The model under review builds one solid part; all positions refer to its coordinate system, in mm. A direction names the side the tool comes from. Round coordinates to 2 decimals unless told otherwise and drop trailing zeros. Loops run counter-clockwise (first coordinate to the right, second up) from the corner with the lowest first, then second, coordinate; pieces in that order, holes last. Notation, with made-up numbers: M -15.75,15 L 27.25,15 A19 cw 27.25,32 Z; hole C 72.5,80.5 d7. An arc over 180 degrees is marked long. One line per question, with ' | ' between items.
from build123d import *

# Parameters (mm, degrees)
BOSS_EXTRUDE1_DEPTH = 5
SKETCH2_R           = 1.5
CUT_EXTRUDE1_DEPTH  = 5


with BuildPart() as part:
    # Sketch1 → Boss-Extrude1 (new body)
    with BuildSketch(Plane(origin=(0, 0, 0), x_dir=(1, 0, 0), z_dir=(0, 1, 0))):
        Polygon((54, 0), (72, 0), (72, -5), (90, -5), (90, 0), (90, 60), (0, 60), (0, 0), (0, -5), (18, -5), (18, 0), (36, 0), (36, -5), (54, -5), align=None)
    extrude(amount=BOSS_EXTRUDE1_DEPTH)

    # Sketch2 → Cut-Extrude1 (cut)
    with BuildSketch(Plane(origin=(0, 5, 0), x_dir=(1, 0, 0), z_dir=(0, 1, 0))):
        with Locations(Location((4.75, 55.25, 0), (0, 0, 270))):
            Circle(SKETCH2_R)
        with Locations(Location((85.25, 55.25, 0), (0, 0, 270))):
            Circle(SKETCH2_R)
        with Locations(Location((85.25, 8.75, 0), (0, 0, 270))):
            Circle(SKETCH2_R)
        with Locations(Location((4.75, 8.75, 0), (0, 0, 270))):
            Circle(SKETCH2_R)
    extrude(amount=-CUT_EXTRUDE1_DEPTH, mode=Mode.SUBTRACT)


solid = part.part
1) Add section D-D on x = 55. State the section outline as (y, z) points.
Output values:
outline: M 0,-60 L 5,-60 L 5,0 L 0,0 Z
2) Add section B-B on x = 4.75. State the section outline as (y, z) points.
Output values:
outline: M 0,-60 L 5,-60 L 5,-56.75 L 0,-56.75 Z; M 0,-53.75 L 5,-53.75 L 5,-10.25 L 0,-10.25 Z; M 0,-7.25 L 5,-7.25 L 5,5 L 0,5 Z
3) Machinability: for faces 1 (the flat face through (54, 2, 3)), 2 (the flat face through (44, 5, -28)), which of the approach directions +Z, -Z, +X, -X, +Y, -Y give a long, thin tool a straight path to every point of the face, cutting with its end or side? Answer none if there is none.
Output values:
face 1: +Z, +Y, -Y | face 2: +Z, -Z, +X, -X, +Y
4) Insertion check: P1, Ø1.5, axis at x = 23, y = 3, coming from the +Z side; P2, Ø1.8, axis at x = 4.75, z = -8.75, coming from the -Y side. Each pin has a flat end and moves straight along its axis. Give the tip position at first contact, or say it passes through.
Output values:
P1: stops at z = 0 | P2: passes through
5) Add section C-C on y = 2.5. State the section outline as (x, z) points.
Output values:
outline: M 0,-60 L 90,-60 L 90,5 L 72,5 L 72,0 L 54,0 L 54,5 L 36,5 L 36,0 L 18,0 L 18,5 L 0,5 Z; hole C 4.75,-55.25 d3; hole C 4.75,-8.75 d3; hole C 85.25,-55.25 d3; hole C 85.25,-8.75 d3
6) For line 1 (Z direction, x = 85.25, y = 3.25); line 2 (X direction, y = 3.05, z = -8.75); line 3 (X direction, y = 1.3, z = 2), list the stretches that pass through material, from the lowest coordinate up.
Output values:
line 1: z = -60 to -56.75, -53.75 to -10.25, -7.25 to 5 | line 2: x = 0 to 3.25, 6.25 to 83.75, 86.75 to 90 | line 3: x = 0 to 18, 36 to 54, 72 to 90
7) Add section A-A on z = -8.75. State the section outline as (x, y) points, then the cut area to 3 significant figures.
Output values:
outline: M 0,0 L 3.25,0 L 3.25,5 L 0,5 Z; M 6.25,0 L 83.75,0 L 83.75,5 L 6.25,5 Z; M 86.75,0 L 90,0 L 90,5 L 86.75,5 Z | area: 420 mm²
